Autodesk Fusion 360 part; units mm, degrees
sketch "Sketch1" plane through (0, 0, 0) normal (0, 0, 1) x (1, 0, 0)
  line L0 (28, -28) -> (-28, -28)
  line L1 (-28, -28) -> (-28, 28)
  line L2 (-28, 28) -> (28, 28)
  line L3 (28, 28) -> (28, -28)
  line L4 (28, -28) -> (-28, 28) construction
  line L5 (-28, -28) -> (28, 28) construction
  dimension "d1" = 56
  dimension "d2" = 56
extrude "Extrude1" add sketch "Sketch1" along normal blind 6
sketch "Sketch2" plane through (28, 0, 0) normal (1, 0, 0) x (0, 1, 0)
  line L0 (-28, 0) -> (28, 0)
  line L1 (28, 0) -> (28, 6)
  line L2 (28, 6) -> (-28, 6)
  line L3 (-28, 6) -> (-28, 0)
  line L4 (-15.0687, 6) -> (1.934, 35.4497)
  line L5 (1.934, 35.4497) -> (13.1924, 28.9497)
  line L6 (13.1924, 28.9497) -> (-0.0576, 6)
  line L7 (7.5632, 32.1997) -> (-7.5632, 6) construction
  line L8 (0, 19.0998) -> (0, 6) construction
  dimension "d5" = 60
  dimension "d6" = 26.5
  dimension "d13" = 13
extrude "Extrude2" add sketch "Sketch2" against normal up to surface (56 mm away) contours L2 L4 L5 L6
sketch "Sketch3" plane through (0, -13.8996, 8.025) normal (0, -0.866, 0.5) x (1, 0, 0)
  line L0 (-28, 31.6673) -> (-28, -2.3382)
  line L1 (-28, -2.3382) -> (28, -2.3382)
  line L2 (28, -2.3382) -> (28, 31.6673)
  line L3 (28, 31.6673) -> (-28, 31.6673)
  line L4 (22.5, 31.6673) -> (22.5, 5.1673)
  line L5 (22.5, 5.1673) -> (0, 5.1673)
  line L6 (0, 5.1673) -> (-22.5, 5.1673)
  line L7 (-22.5, 5.1673) -> (-22.5, 31.6673)
  line L8 (0, -2.3382) -> (0, 5.1673) construction
  dimension "d9" = 45
  dimension "d10" = 26.5
extrude "Extrude3" cut sketch "Sketch3" against normal up to surface (13 mm away) contours L3 L4 L5 L6 L7
sketch "Sketch4" plane through (0, 15.8337, 27.4247) normal (0, 0.5, 0.866) x (-1, 0, 0)
  line L0 (22.5, 16.0499) -> (22.5, 3.0499)
  line L1 (22.5, 3.0499) -> (28, 3.0499)
  line L2 (28, 3.0499) -> (28, 16.0499)
  line L3 (28, 16.0499) -> (22.5, 16.0499)
  line L4 (22.5, 11.0499) -> (24, 11.0499) construction
  line L5 (24, 11.0499) -> (22.5, 3.0499)
  line L6 (24, 11.0499) -> (22.5, 16.0499)
  line L7 (-24, 11.0499) -> (-22.5, 16.0499)
  line L8 (-24, 11.0499) -> (-22.5, 3.0499)
  line L9 (-22.5, 3.0499) -> (-22.5, 16.0499)
  line L10 (-22.5, 11.0499) -> (-24, 11.0499) construction
  line L11 (22.5, 9.5499) -> (-22.5, 9.5499) construction
  line L12 (22.5, 11.0499) -> (-22.5, 11.0499) construction
  point P0 (-22.5, 16.0499)
  point P1 (-22.5, 3.0499)
  dimension "d27" = 48
  dimension "d29" = 1.5
extrude "Extrude4" cut sketch "Sketch4" against normal up to surface (27 mm away) from surface at -9.5 contours L0 L5 L6 | L7 L8 L9
sketch "Sketch5" plane through (0, 0, 6) normal (0, 0, 1) x (-1, 0, 0)
  line L0 (28, -28) -> (28, 0.0576)
  line L1 (28, 0.0576) -> (22.5, 0.0576)
  line L2 (-28, 0.0576) -> (-28, -28)
  line L3 (-28, -28) -> (28, -28)
  line L4 (-23, 0.0576) -> (-23, -23)
  line L5 (-23, -23) -> (0, -23)
  line L6 (0, -23) -> (23, -23)
  line L7 (23, 0.0576) -> (23, -23)
  line L8 (0, 0) -> (0, -23) construction
  line L9 (-28, 15.0687) -> (28, 15.0687)
  line L10 (23, 0.0576) -> (23, 15.0687) construction
  line L11 (-23, 0.0576) -> (-23, 15.0687) construction
  line L12 (-23, 15.0687) -> (-23, 23)
  line L13 (-23, 23) -> (23, 23)
  line L14 (23, 15.0687) -> (23, 23)
  line L15 (-23, 23) -> (-23, 28) construction
  line L16 (28, 28) -> (-28, 28) construction
  line L17 (-23, -23) -> (-23, -28) construction
  line L18 (-23, -23) -> (-28, -23) construction
  line L19 (22.5, 0.0576) -> (-22.5, 0.0576)
  line L20 (-22.5, 0.0576) -> (-28, 0.0576)
  dimension "d24" = 5
extrude "Extrude5" cut sketch "Sketch5" against normal through all contours L1 L4 L5 L6 L7 L19 L20 | L9 L12 L13 L14
fillet "Fillet1" radius 5 8 edges at (28, 28, 3) (-28, 28, 3) (28, -28, 3) (-28, -28, 3) (23, 23, 3) (-23, 23, 3) (23, -23, 3) (-23, -23, 3)
fillet "Fillet2" radius 5 4 edges at (28, -6.5674, 20.7248) (28, 6.5674, 17.4748) (-28, -6.5674, 20.7248) (-28, 6.5674, 17.4748)
sketch "Sketch6" plane through (0, 0, 0) normal (0, 0, -1) x (1, 0, 0)
  arc A0 (-23, 28) -> (-28, 23) centre (-23, 23) ccw
  line L0 (-28, 23) -> (-28, -23)
  arc A1 (-28, -23) -> (-23, -28) centre (-23, -23) ccw
  line L1 (-23, -28) -> (23, -28)
  arc A2 (23, -28) -> (28, -23) centre (23, -23) ccw
  line L2 (28, -23) -> (28, 23)
  arc A3 (28, 23) -> (23, 28) centre (23, 23) ccw
  line L3 (23, 28) -> (-23, 28)
  line L4 (-23, -18) -> (-23, 0.0576)
  line L5 (-23, 0.0576) -> (23, 0.0576)
  line L6 (23, 0.0576) -> (23, -18)
  arc A4 (18, -23) -> (23, -18) centre (18, -18) ccw
  line L7 (18, -23) -> (-18, -23)
  arc A5 (-23, -18) -> (-18, -23) centre (-18, -18) ccw
  line L8 (23, 18) -> (23, 15.0687)
  line L9 (23, 15.0687) -> (-23, 15.0687)
  line L10 (-23, 15.0687) -> (-23, 18)
  arc A6 (-18, 23) -> (-23, 18) centre (-18, 18) ccw
  line L11 (-18, 23) -> (18, 23)
  arc A7 (23, 18) -> (18, 23) centre (18, 18) ccw
  line L12 (-23, 0.0576) -> (23, 0.0576)
  line L13 (23, 15.0687) -> (-23, 15.0687)
  line L14 (20, 0.0576) -> (20, 15.0687)
  line L15 (-20, 15.0687) -> (-20, 0.0576)
  line L16 (20, 7.5632) -> (0, 7.5632) construction
  line L17 (0, 7.5632) -> (0, 0) construction
  line L18 (0, 7.5632) -> (-20, 7.5632) construction
  dimension "d25" = 3
extrude "Extrude6" cut sketch "Sketch6" against normal through all contours L5 L9 L12 L13 L14 L15
chamfer "Chamfer1" distance 1.45 angle 45 4 edges at (23.25, 4.9783, 22.7224) (23.25, -0.6509, 25.9724) (-23.25, 4.9783, 22.7224) (-23.25, -0.6509, 25.9724)
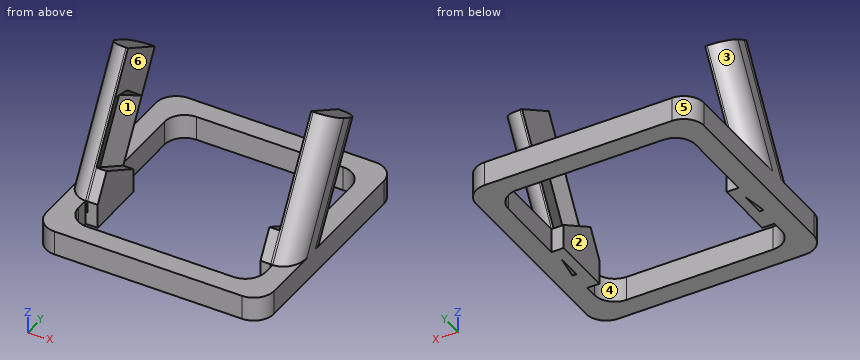
Build history of the part. All positions in model axes, mm. Face numbers are marked on the shaded views. A direction names the side the tool comes from. Coordinates: 2 decimals unless noted, no trailing zeros. Write each loop counter-clockwise with the first axis right and the second up, starting at its lowest first coordinate (ties: lowest second). Pieces come first, ordered by that corner, then holes.
(1) Drill centre lines: line 1 (Y direction, x = 13, z = 2); line 2 (Z direction, x = -25, y = -18); line 3 (Y direction, x = -19.5, z = 1.5). Where is each one in solid material? Low to high.
(2) Pin check, flat tips, straight feed: pin 1 Ø5 at (y, z) = (1, 24.5) entering from +X; pin 2 Ø8 at (y, z) = (-9.5, 16) entering from -X; pin 3 Ø10 at (x, y) = (10.5, 15.5) entering from +Z; pin 4 Ø10 at (x, z) = (-20, 28) entering from +Y. Stop position of each tip, or through.
(3) 3-axis set-ups, long thin cutter, end or side, ignore diameter. For the marked faces 1, 2 and 3: which of +Z, -Z, +X, -X, +Y, -Y reach the whole face in a straight line?
(4) Mould opens along Y. For the marked faces 4, 5 and 6 say: pulls with the +Y half, pulls with the -Y half, needs draft (parallel to the pull), parting line crosses it, or undercut.
(5) Cut at A-A on x = -5.5. List the corners of the cut face in (y, z).
(6) Cut at C-C on y = 20. List the corners of the cut face in (x, z).
Working result:
1. line 1: y = -28 to -23, 23 to 28
1. line 2: z = 0 to 6
1. line 3: y = -28 to -22.77, 22.77 to 28
2. pin 1: stops at x = 28
2. pin 2: stops at x = -27.86
2. pin 3: passes through
2. pin 4: stops at y = 13.19
3. face 1: none
3. face 2: +Z, -Z
3. face 3: -X, +Y
4. face 4: undercut
4. face 5: pulls with the +Y half
4. face 6: needs draft
5. outline: (-28, 0) - (-23, 0) - (-23, 6) - (-28, 6) - close; (23, 0) - (28, 0) - (28, 6) - (23, 6) - close
6. outline: (-28, 0) - (-22.58, 0) - (-22.58, 6) - (-28, 6) - close; (22.58, 0) - (28, 0) - (28, 6) - (22.58, 6) - close
